```python
from build123d import *

# Parameters (mm, degrees)
SKETCH1_W           = 20
SKETCH1_H           = 4
SKETCH1_W_2         = 4
SKETCH1_H_2         = 20
BOSS_EXTRUDE1_DEPTH = 20
SKETCH2_R           = 2.125
CUT_EXTRUDE1_DEPTH  = 100.735876193
SKETCH3_R           = 2.125
CUT_EXTRUDE2_DEPTH  = 108.560738655
CHAMFER1_SIZE       = 2
CHAMFER2_SIZE       = 2.5
FILLET1_R           = 1


with BuildPart() as part:
    # Sketch1 → Boss-Extrude1 (new body)
    with BuildSketch(Plane.XY):
        with Locations((-16, -11.85)):
            Rectangle(SKETCH1_W, SKETCH1_H)
        Polygon((58.65, 48.3), (58.65, 42.3), (0, 42.3), (0, -13.85), (-6, -13.85), (-6, 48.3), align=None)
        with Locations((56.65, 58.3)):
            Rectangle(SKETCH1_W_2, SKETCH1_H_2)
    extrude(amount=BOSS_EXTRUDE1_DEPTH)

    # Sketch2 → Cut-Extrude1 (cut, through all)
    with BuildSketch(Plane(origin=(0, -9.85, 0), x_dir=(1, 0, 0), z_dir=(0, 1, 0))):
        with Locations(Location((-16, -10, 0), (0, 0, 180))):
            Circle(SKETCH2_R)
    extrude(amount=-CUT_EXTRUDE1_DEPTH, mode=Mode.SUBTRACT)

    # Sketch3 → Cut-Extrude2 (cut, through all)
    with BuildSketch(Plane.ZY.offset(-54.65)):
        with Locations(Location((10, 58.3, 0), (0, 0, 270))):
            Circle(SKETCH3_R)
    extrude(amount=-CUT_EXTRUDE2_DEPTH, mode=Mode.SUBTRACT)

    # Chamfer1
    chamfer1_edges = [part.edges().sort_by_distance(p)[0] for p in [
        (-13.875, -9.85, 10),
        (54.65, 60.425, 10),
    ]]
    chamfer(chamfer1_edges, length=CHAMFER1_SIZE)

    # Chamfer2
    chamfer2_edges = [part.edges().sort_by_distance(p)[0] for p in [
        (-6, -9.85, 10),
        (54.65, 48.3, 10),
    ]]
    chamfer(chamfer2_edges, length=CHAMFER2_SIZE)

    # Fillet1
    fillet1_edges = [part.edges().sort_by_distance(p)[0] for p in [
        (-6, 48.3, 10),
        (0, 42.3, 10),
    ]]
    fillet(fillet1_edges, radius=FILLET1_R)


solid = part.part
```
The listing builds one solid part. Answer for the finished solid, in the listing's coordinates (mm). A direction names the side the tool comes from. Coordinates: 2 decimals unless noted, no trailing zeros. Write each loop counter-clockwise with the first axis right and the second up, starting at its lowest first coordinate (ties: lowest second). Pieces come first, ordered by that corner, then holes. Notation, with made-up numbers: (-16.75, 65.25) - (-10.75, 65.25) arc R19 cw to (-10.75, 81.25) - close; hole circle Ø6 at (17.25, -39). An arc over 180 degrees is marked (long way). Return JSON: item names as keys, results as strings. Group by question number.
Q1. For a pull along Z with two mould halves and no side action, classify faces 4 (the flat face through (13, 43, 0)), 5 (the cylindrical face through (57.636, 56.273, 10.638)), 6 (the flat face through (30, 42.3, 10)) as +Z half, -Z half, draft (parallel to the pull), parting line (faces both ways), or undercut.
Q2. The part is cut by section A-A on x = -16. Write down the section's boundary in (y, z) (3 decimals), and give its area (3 significant figures).
Q3. The part is cut by section B-B on y = 58.3. Write down the section's boundary in (x, z) (3 decimals), and give its area (3 significant figures).
Q4. The part is cut by section C-C on z = 10. Write down the section's boundary in (x, y) (3 decimals).
Q5. Find the intervals of material crossed by line 1 along Z through (x, y) = (-16, -12) (3 decimals); line 2 along X through (y, z) = (3.5, 3.5); line 3 along Y through (x, z) = (14.5, 1.5), in increasing order. Write a range as [from, to].
Q6. Which of the six approach directions +Z, -Z, +X, -X, +Y, -Y give full straight-line access (tool end or side, diameter ignored) to faces 1 (the flat face through (-26, -12, 10)), 2 (the flat face through (-6, 20, 10)), 3 (the flat face through (0, 14, 10))?
Q7. The part is cut by section D-D on z = 16. Write down the section's boundary in (x, y).
Q8. Flat-ended cylindrical pins translate along their axes: pin 1 Ø3 at (y, z) = (29.5, 3) entering from -X; pin 2 Ø10 at (x, z) = (26, 5) entering from -Y; pin 3 Ø6 at (x, z) = (18, 14.5) entering from +Y; pin 4 Ø5 at (x, z) = (-16, 10) entering from -Y. Find the tip coordinate at first contact, or state that the pin passes through.
Evaluation:
{
 "1": {"face 4": "-Z half", "face 5": "undercut", "face 6": "draft"},
 "2": {"outline": "(-13.85, 0) - (-9.85, 0) - (-9.85, 5.875) - (-11.85, 7.875) - (-13.85, 7.875) - close; (-13.85, 12.125) - (-11.85, 12.125) - (-9.85, 14.125) - (-9.85, 20) - (-13.85, 20) - close", "area": "59.0 mm2"},
 "3": {"outline": "(54.65, 0) - (58.65, 0) - (58.65, 7.875) - (56.65, 7.875) - (54.65, 5.875) - close; (54.65, 14.125) - (56.65, 12.125) - (58.65, 12.125) - (58.65, 20) - (54.65, 20) - close", "area": "59.0 mm2"},
 "4": {"outline": "(-26, -13.85) - (-18.125, -13.85) - (-18.125, -11.85) - (-20.125, -9.85) - (-26, -9.85) - close; (-13.875, -13.85) - (0, -13.85) - (0, 41.3) arc R1 cw to (1, 42.3) - (58.65, 42.3) - (58.65, 56.175) - (56.65, 56.175) - (54.65, 54.175) - (54.65, 50.8) - (52.15, 48.3) - (-5, 48.3) arc R1 ccw to (-6, 47.3) - (-6, -7.35) - (-8.5, -9.85) - (-11.875, -9.85) - (-13.875, -11.85) - close; (54.65, 62.425) - (56.65, 60.425) - (58.65, 60.425) - (58.65, 68.3) - (54.65, 68.3) - close"},
 "5": {"line 1": "z = [0, 7.875], [12.125, 20]", "line 2": "x = [-6, 0]", "line 3": "y = [42.3, 48.3]"},
 "6": {"face 1": "+Z, -Z, -X, +Y, -Y", "face 2": "+Z, -Z, -X, +Y", "face 3": "+Z, -Z, +X, -Y"},
 "7": {"outline": "(-26, -13.85) - (0, -13.85) - (0, 41.3) arc R1 cw to (1, 42.3) - (58.65, 42.3) - (58.65, 68.3) - (54.65, 68.3) - (54.65, 50.8) - (52.15, 48.3) - (-5, 48.3) arc R1 ccw to (-6, 47.3) - (-6, -7.35) - (-8.5, -9.85) - (-26, -9.85) - close"},
 "8": {"pin 1": "stops at x = -6", "pin 2": "stops at y = 42.3", "pin 3": "stops at y = 48.3", "pin 4": "stops at y = -13.85"}
}
